For this review, take the finished solid that the model builds, in its own axes (mm). Coordinates: 2 decimals unless noted, no trailing zeros. Write each loop counter-clockwise with the first axis right and the second up, starting at its lowest first coordinate (ties: lowest second). Pieces come first, ordered by that corner, then holes.
1) We need section C-C on y = -8.5. Give the number of separate pieces and of enclosed holes in the cut face, then the cut area to 3 significant figures.
2) We need section D-D on x = 22. Write out the cut boundary in (y, z), then the cut area to 3 significant figures.
3) We need section A-A on z = 6. Write out the cut boundary in (x, y).
4) To check wall thickness, follow line 1 along Z through (x, y) = (0, 7.35); line 2 along X through (y, z) = (0, -9); line 3 along X through (y, z) = (-2.75, 15). State the ranges of each line that lie inside material, in increasing order.
5) Insertion check: P1, Ø3, axis at x = -22, z = 0, coming from the -Y side; P2, Ø1, axis at y = -1.5, z = -20.5, coming from the -X side; P3, Ø5, axis at y = -3.5, z = 20.5, coming from the +X side; P4, Ø2, axis at y = -4, z = -18.5, coming from the +X side. Each pin has a flat end and moves straight along its axis. Give the tip position at first contact, or say it passes through.
6) We need section B-B on y = -2. Write out the cut boundary in (x, z), then the cut area to 3 significant figures.
7) Mouldability with a two-part tool opening along Y and no side actions: class faces 1 (the face through (0, 10, 0)), 2 (the face through (-16.887, -0.14, -14.864)), 3 (the face through (0, -10, 0)), 4 (the face through (-13, 0, 5)) as pulls with the +Y half, pulls with the -Y half, needs draft (parallel to the pull), parting line crosses it, or undercut.
from build123d import *

# Parameters (mm, degrees)
SKETCH1_R           = 1.25
SKETCH1_R_2         = 1.5
BOSS_EXTRUDE1_DEPTH = 10
CUT_EXTRUDE4_REACH  = 63.196
SKETCH7_R           = 5
CUT_EXTRUDE5_REACH  = 63.196
SKETCH8_R           = 5


with BuildPart() as part:
    # Sketch1 → Boss-Extrude1 (new, symmetric)
    with BuildSketch(Plane(origin=(0, 0, 0), x_dir=(1, 0, 0), z_dir=(0, 1, 0))):
        Polygon((11.183766184, 27), (-11.183766184, 27), (-27, 11.183766184), (-27, -11.183766184), (-11.183766184, -27), (11.183766184, -27), (27, -11.183766184), (27, 11.183766184), align=None)
        with Locations(Location((0, 22, 0), (0, 0, 270))):
            Circle(SKETCH1_R, mode=Mode.SUBTRACT)
        with Locations(Location((15.556349186, 15.556349186, 0), (0, 0, 270))):
            Circle(SKETCH1_R_2, mode=Mode.SUBTRACT)
        with Locations(Location((22, 0, 0), (0, 0, 270))):
            Circle(SKETCH1_R, mode=Mode.SUBTRACT)
        with Locations(Location((15.556349186, -15.556349186, 0), (0, 0, 270))):
            Circle(SKETCH1_R_2, mode=Mode.SUBTRACT)
        with Locations(Location((0, -22, 0), (0, 0, 270))):
            Circle(SKETCH1_R, mode=Mode.SUBTRACT)
        with Locations(Location((-15.556349186, -15.556349186, 0), (0, 0, 270))):
            Circle(SKETCH1_R_2, mode=Mode.SUBTRACT)
        with Locations(Location((-22, 0, 0), (0, 0, 270))):
            Circle(SKETCH1_R, mode=Mode.SUBTRACT)
        with Locations(Location((-15.556349186, 15.556349186, 0), (0, 0, 270))):
            Circle(SKETCH1_R_2, mode=Mode.SUBTRACT)
    extrude(amount=BOSS_EXTRUDE1_DEPTH, both=True)

    # Cut-Extrude4: up to this face of the body (flat: up to its plane)
    cut_extrude4_end = Plane(part.part.faces().sort_by_distance((0, 0, -27))[0])
    # Sketch7 → Cut-Extrude4 (cut, up to the picked face)
    with BuildSketch(Plane.XY.offset(27), mode=Mode.PRIVATE) as cut_extrude4_sk1:
        Circle(SKETCH7_R)
    cut_extrude4_tool1 = split(extrude(cut_extrude4_sk1.sketch, amount=-CUT_EXTRUDE4_REACH, mode=Mode.PRIVATE), bisect_by=cut_extrude4_end, keep=Keep.BOTH, mode=Mode.PRIVATE)
    add(cut_extrude4_tool1.solids().sort_by(Axis((0, 0, 27), (0, 0, -1)))[0], mode=Mode.SUBTRACT)

    # Cut-Extrude5: up to this face of the body (flat: up to its plane)
    cut_extrude5_end = Plane(part.part.faces().sort_by_distance((-27, 0, 0))[0])
    # Sketch8 → Cut-Extrude5 (cut, up to the picked face)
    with BuildSketch(Plane(origin=(27, 0, 0), x_dir=(0, 0, -1), z_dir=(1, 0, 0)), mode=Mode.PRIVATE) as cut_extrude5_sk1:
        Circle(SKETCH8_R)
    cut_extrude5_tool1 = split(extrude(cut_extrude5_sk1.sketch, amount=-CUT_EXTRUDE5_REACH, mode=Mode.PRIVATE), bisect_by=cut_extrude5_end, keep=Keep.BOTH, mode=Mode.PRIVATE)
    add(cut_extrude5_tool1.solids().sort_by(Axis((27, 0, 0), (-1, 0, 0)))[0], mode=Mode.SUBTRACT)


solid = part.part
Result:
1. separate pieces: 1
1. enclosed holes: 8
1. area: 2,370 mm2
2. outline: (-10, -16.18) - (10, -16.18) - (10, -1.25) - (4.84, -1.25) arc R5 cw to (-4.84, -1.25) - (-10, -1.25) - close; (-10, 1.25) - (-4.84, 1.25) arc R5 cw to (4.84, 1.25) - (10, 1.25) - (10, 16.18) - (-10, 16.18) - close
2. area: 544 mm2
3. outline: (-27, -10) - (27, -10) - (27, 10) - (-27, 10) - close; hole circle Ø10 at (0, 0)
4. line 1: z = -27 to -23.25, -20.75 to 20.75, 23.25 to 27
4. line 2: x = -27 to -5, 5 to 27
4. line 3: x = -23.18 to -16.95, -14.16 to -4.18, 4.18 to 14.16, 16.95 to 23.18
5. P1: stops at y = -10
5. P2: stops at x = -18.18
5. P3: stops at x = 20.18
5. P4: stops at x = 20.68
6. outline: (-27, -11.18) - (-11.18, -27) - (-4.58, -27) - (-4.58, -4.58) - (-27, -4.58) - close; (-27, 4.58) - (-4.58, 4.58) - (-4.58, 27) - (-11.18, 27) - (-27, 11.18) - close; (4.58, -27) - (11.18, -27) - (27, -11.18) - (27, -4.58) - (4.58, -4.58) - close; (4.58, 4.58) - (27, 4.58) - (27, 11.18) - (11.18, 27) - (4.58, 27) - close; hole circle Ø3 at (-15.56, -15.56); hole circle Ø3 at (-15.56, 15.56); hole circle Ø3 at (15.56, -15.56); hole circle Ø3 at (15.56, 15.56)
6. area: 1,480 mm2
7. face 1: pulls with the +Y half
7. face 2: needs draft
7. face 3: pulls with the -Y half
7. face 4: undercut
